Verification items for the finished model (mm, model axes). Face numbers are marked on the shaded views. A direction names the side the tool comes from. Give positions to 0.01 mm unless a question says otherwise; leave off trailing zeros. Write each loop counter-clockwise with the first axis right and the second up, starting at its lowest first coordinate (ties: lowest second). Pieces come first, ordered by that corner, then holes. Notation, with made-up numbers: (14.25, 24) - (62.25, 24) arc R24 ccw to (62.25, 44) - close; hole circle Ø2 at (8, -9). An arc over 180 degrees is marked (long way). Answer as a JSON object with one key per item and string values. Group by question number.
Item 1: Sectioned sample at D-D, the plane x = 19. Record the boundary of the cut face in (y, z).
Item 2: Sectioned sample at B-B, the plane x = -1. Record the boundary of the cut face in (y, z).
Item 3: Sectioned sample at C-C, the plane z = -2. Record the boundary of the cut face in (x, y), and give its area (3 significant figures).
Item 4: Scan lines: line 1 along X through (y, z) = (-0.5, 10); line 2 along Z through (x, y) = (-25.5, 3.5); line 3 along Y through (x, z) = (-18.5, -1.5). Record each from-to range of solid material in increasing order. Write a range as [from, to].
Item 5: Go/stop test with flat-tipped pins: pin 1 (6 mm diameter, centred on x = 18, z = 10, fed in from -Y); pin 2 (1.5 mm diameter, centred on y = -0.5, z = 11.5, fed in from +X); pin 3 (2 mm diameter, centred on y = 3.5, z = 5, fed in from -X); pin 4 (1.5 mm diameter, centred on y = -0.5, z = -8.5, fed in from -X). Record where each tip stops, or that it passes through.
Item 6: Tool access check on the marked faces 1, 2 and 3. Record the directions out of +Z, -Z, +X, -X, +Y, -Y that give a thin tool (end or side, any length) a straight path to the whole face; none if there is none.
Item 7: Sectioned sample at A-A, the plane y = 0. Record the boundary of the cut face in (x, z), and give its area (3 significant figures).
```python
from build123d import *

# Parameters (mm, degrees)
SKETCH_1_W = 80
SKETCH_1_H = 5
SKETCH_2_W = 5
SKETCH_2_H = 60


with BuildPart() as part:
    # 草图1 → 旋转1 (revolve)
    with BuildSketch(Plane.XY, mode=Mode.PRIVATE) as revolve_1_sk:
        with Locations((0, 2.5)):
            Rectangle(SKETCH_1_W, SKETCH_1_H)
    revolve(revolve_1_sk.sketch.rotate(Axis((-40, 0, 0), (1, 0, 0)), 90), axis=Axis((-40, 0, 0), (1, 0, 0)))

    # 草图2 → 旋转2 (revolve)
    with BuildSketch(Plane(origin=(0, 0, 0), x_dir=(1, 0, 0), z_dir=(0, 1, 0))):
        with Locations((2.5, 0)):
            Rectangle(SKETCH_2_W, SKETCH_2_H)
    revolve(axis=Axis((0, 0, 30), (0, 0, -1)))


solid = part.part
```
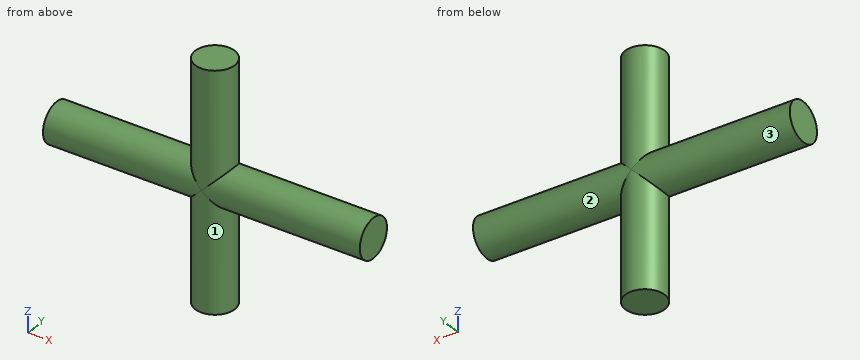
Geometry check:
{
 "1": {"outline": "circle Ø10 at (0, 0)"},
 "2": {"outline": "(-4.9, -30) - (4.9, -30) - (4.9, -1) arc R5 ccw to (4.9, 1) - (4.9, 30) - (-4.9, 30) - (-4.9, 1) arc R5 ccw to (-4.9, -1) - close"},
 "3": {"outline": "(-40, -4.58) - (-2, -4.58) arc R5 ccw to (2, -4.58) - (40, -4.58) - (40, 4.58) - (2, 4.58) arc R5 ccw to (-2, 4.58) - (-40, 4.58) - close", "area": "735 mm^2"},
 "4": {"line 1": "[-4.97, 4.97]", "line 2": "[-3.57, 3.57]", "line 3": "[-4.77, 4.77]"},
 "5": {"pin 1": "through", "pin 2": "x = 5", "pin 3": "x = -4.33", "pin 4": "x = -5"},
 "6": {"face 1": "-Z", "face 2": "+X", "face 3": "-X"},
 "7": {"outline": "(-40, -5) - (-5, -5) - (-5, -30) - (5, -30) - (5, -5) - (40, -5) - (40, 5) - (5, 5) - (5, 30) - (-5, 30) - (-5, 5) - (-40, 5) - close", "area": "1,300 mm^2"}
}
